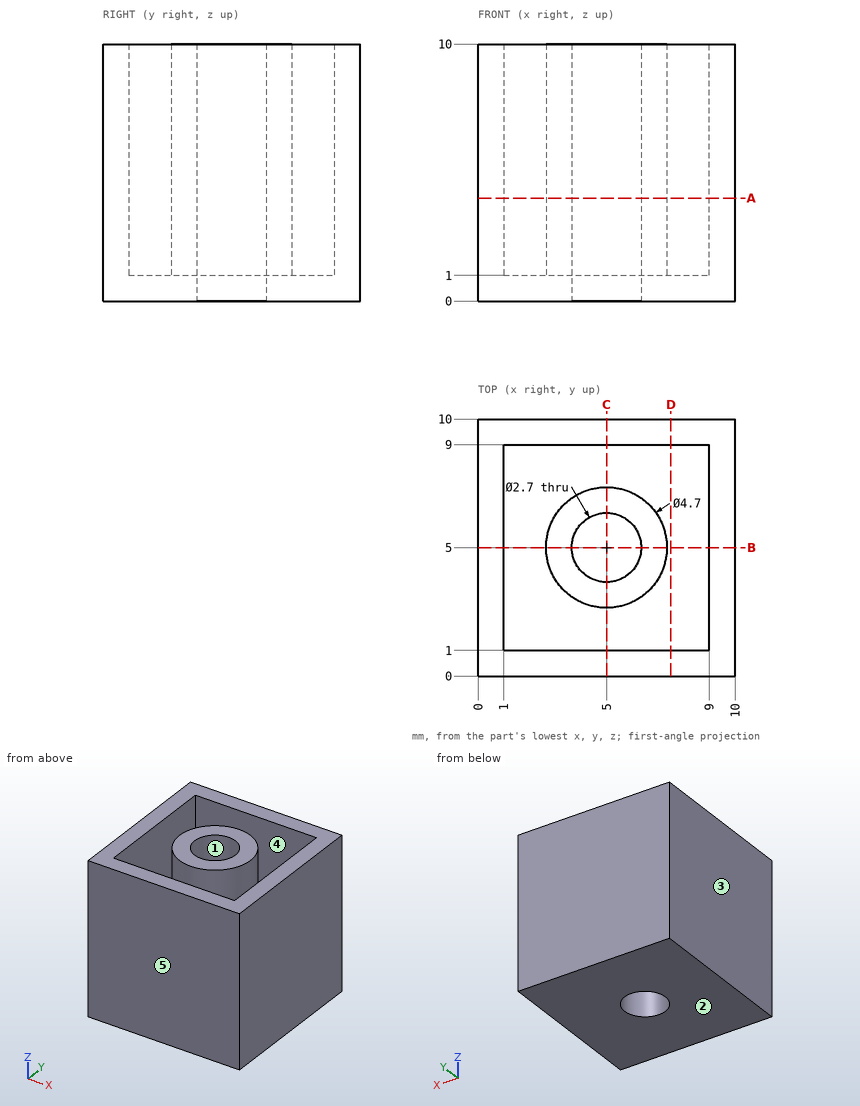
Geometry: see drawing. Coordinates: mm, zero at the bounding-box minimum. A direction names the side the tool comes from. Give positions to 0.01 mm unless a question says otherwise; leave off trailing zeros. Write each loop counter-clockwise with the first axis right and the second up, starting at its lowest first coordinate (ties: lowest second). Pieces come first, ordered by that corner, then holes. Notation, with made-up numbers: M -17.75,85 L -5.75,85 A16 ccw -5.75,107 Z; hole C 40,14.5 d2. An arc over 180 degrees is marked long. Answer as a JSON object with one key per item and string values.
Q1. Contact query for a flat-ended pin moving along its axis: P1, Ø1, axis at y = 9, z = 8, coming from the -X side. Output: stop coordinate, or through.
Geometry check:
{"P1": "stops at x = 0"}
Q2. Access query for the marked faces 4 and 5. Directions: +Z, -Z, +X, -X, +Y, -Y. A direction counts if a zero-diameter tool reaches every point of the face in a straight line with its end or side. Return the directions, or none.
Geometry check:
{"face 4": "+Z", "face 5": "+Z, -Z, +X, -X, -Y"}
Q3. Ray query, line 1 along Y through (x, z) = (5, 3.25); line 2 along Y through (x, z) = (1.75, 8.5); line 3 along X through (y, z) = (4, 4.5). Return the intervals inside material, ascending.
Geometry check:
{"line 1": "y = 0 to 1, 2.65 to 3.65, 6.35 to 7.35, 9 to 10", "line 2": "y = 0 to 1, 9 to 10", "line 3": "x = 0 to 1, 2.87 to 4.09, 5.91 to 7.13, 9 to 10"}
Q4. Cut plane B-B, the plane y = 5. Return the cut outline in (x, z).
Geometry check:
{"outline": "M 0,0 L 3.65,0 L 3.65,10 L 2.65,10 L 2.65,1 L 1,1 L 1,10 L 0,10 Z; M 6.35,0 L 10,0 L 10,10 L 9,10 L 9,1 L 7.35,1 L 7.35,10 L 6.35,10 Z"}
Q5. Cut plane D-D, the plane x = 7.5. Return the cut outline in (y, z).
Geometry check:
{"outline": "M 0,0 L 10,0 L 10,10 L 9,10 L 9,1 L 1,1 L 1,10 L 0,10 Z"}
Q6. Cut plane A-A, the plane z = 4. Return the cut outline in (x, y).
Geometry check:
{"outline": "M 0,0 L 10,0 L 10,10 L 0,10 Z; C 5,5 d4.7; hole M 1,1 L 9,1 L 9,9 L 1,9 Z; hole C 5,5 d2.7"}
Q7. Mould query, pull axis X, two halves, no side actions, for the marked faces 1, 2 and 3. Classes: +X half, -X half, draft (parallel to the pull), parting line (faces both ways), or undercut.
Geometry check:
{"face 1": "undercut", "face 2": "draft", "face 3": "-X half"}
